Could you check a few things on this model? Use its own coordinates, in mm. A direction names the side the tool comes from. Give positions to 0.01 mm unless a question says otherwise; leave off trailing zeros. Order: outer loops, then holes, each group sorted by start corner. A loop starts at its lowest first (then second) coordinate and runs counter-clockwise, first axis right, second up. Notation, with made-up numbers: M 81.25,8 L 128.25,8 A32 ccw 128.25,37 Z; hole C 48,38 d6. An arc over 180 degrees is marked long. Use a Markdown table: item, result. Add a question column.
Item 1: I'm going to push flat-ended pins straight in: pin 1 Ø9 at (x, z) = (8, 5.5) entering from +Y; pin 2 Ø1 at (x, z) = (14, 11) entering from +Y; pin 3 Ø3.5 at (y, z) = (9.5, 13) entering from -X; pin 4 Ø8.5 at (x, z) = (8.5, 4) entering from -Y. Where does each tip first touch, or does it pass through?
Item 2: If I drill on L1, parallel to Y at x = 11, z = 3.25; L2, parallel to Z at x = 6, y = 9.75; L3, parallel to X at y = 2.75, z = 8.5, over which ranges is the centre line in solid material (lowest first)? Write a range as from..to.
Item 3: If we mould it in two halves opening along Y, with no side actions, what happens to faces 4 (the face through (6, 5, 27)), 5 (the face through (-0.25, 1, 13)), 6 (the face through (0, 6.65, 13))? For each: released by +Y, released by -Y, zero draft, split by the parting line, or undercut.
Item 4: For faces 1 (the face through (2.4, 7.22, 13.79)), 2 (the face through (6, 4.65, 13)), 3 (the face through (6, -2.15, 4)), which set-ups out of +Z, -Z, +X, -X, +Y, -Y let a thin tool reach every point of the face, with its end or its side?
Item 5: Suppose I cut it at D-D on z = 3.5. Write out the boundary of the cut face in (x, y).
Item 6: Suppose I cut it at A-A on x = 6. Write out the boundary of the cut face in (y, z), plus the area to 3 significant figures.
Item 7: Suppose I cut it at B-B on z = 23.5. Write out the boundary of the cut face in (x, y), plus the area to 3 significant figures.
Item 8: Suppose I cut it at C-C on y = 1.25. Write out the boundary of the cut face in (x, z).
from build123d import *

# Parameters (mm, degrees)
F0_W      = 12.5
F0_H      = 4.8
F1_DEPTH  = 27
F2_W      = 12.5
F2_H      = 6.8
F3_DEPTH  = 19
F4_W      = 1.5
F4_H      = 0.3
F5_DEPTH  = 3
F6_R      = 1.3
F7_DEPTH  = 13.801
F8_R      = 2
F10_DEPTH = 0.2


with BuildPart() as f1:
    # F0 (on Top) → F1 (new body)
    with BuildSketch(Plane.XY):
        Polygon((3, 6.65), (-2.25, 6.65), (-2.25, -2.15), (14.25, -2.15), (14.25, 6.65), (9, 6.65), (9, 11.65), (3, 11.65), align=None)
        with Locations((6, 2.25)):
            Rectangle(F0_W, F0_H, mode=Mode.SUBTRACT)
    extrude(amount=F1_DEPTH)

    # F2 (on face) → F3 (cut)
    with BuildSketch(Plane.XY.offset(27)):
        with Locations((6, 1.25)):
            Rectangle(F2_W, F2_H)
    extrude(amount=-F3_DEPTH, mode=Mode.SUBTRACT)

    # F4 (on face) → F5 (join)
    with BuildSketch(Plane.XY.offset(8)):
        with Locations((0.5, 0)):
            Rectangle(F4_W, F4_H)
        with Locations((11.5, 0)):
            Rectangle(F4_W, F4_H)
    extrude(amount=-F5_DEPTH)

    # F6 (on face) → F7 (cut, through all)
    with BuildSketch(Plane(origin=(0, 11.65, 0), x_dir=(-1, 0, 0), z_dir=(0, 1, 0))):
        with Locations((-6, 23.5)):
            Circle(F6_R)
    extrude(amount=-F7_DEPTH, mode=Mode.SUBTRACT)

    # F8
    f8_edges = [f1.edges().sort_by_distance(p)[0] for p in [
        (9, 6.65, 13.5),
        (3, 6.65, 13.5),
        (-2.25, 6.65, 13.5),
        (-2.25, -2.15, 13.5),
        (14.25, 6.65, 13.5),
        (14.25, -2.15, 13.5),
        (6, 11.65, 27),
    ]]
    fillet(f8_edges, radius=F8_R)

    # F9 (on face) → F10 (join)
    with BuildSketch(Plane(origin=(0, 0, 0), x_dir=(1, 0, 0), z_dir=(0, 0, -1))):
        with BuildLine():
            ThreePointArc((-0.25, 4.15), (-3.0784271247, 2.9784271247), (-4.25, 0.15))
            Line((-4.25, 0.15), (-4.25, -4.65))
            ThreePointArc((-4.25, -4.65), (-3.0784271247, -7.4784271247), (-0.25, -8.65))
            Line((-0.25, -8.65), (1, -8.65))
            Line((1, -8.65), (1, -11.65))
            ThreePointArc((1, -11.65), (1.5857864376, -13.0642135624), (3, -13.65))
            Line((3, -13.65), (9, -13.65))
            ThreePointArc((9, -13.65), (10.4142135624, -13.0642135624), (11, -11.65))
            Line((11, -11.65), (11, -8.65))
            Line((11, -8.65), (12.25, -8.65))
            ThreePointArc((12.25, -8.65), (15.0784271247, -7.4784271247), (16.25, -4.65))
            Line((16.25, -4.65), (16.25, 0.15))
            ThreePointArc((16.25, 0.15), (15.0784271247, 2.9784271247), (12.25, 4.15))
            Line((12.25, 4.15), (-0.25, 4.15))
        make_face()
        with BuildLine():
            ThreePointArc((-0.25, -6.65), (-1.6642135624, -6.0642135624), (-2.25, -4.65))
            Line((-2.25, -4.65), (-2.25, 0.15))
            ThreePointArc((-2.25, 0.15), (-1.6642135624, 1.5642135624), (-0.25, 2.15))
            Line((-0.25, 2.15), (12.25, 2.15))
            ThreePointArc((12.25, 2.15), (13.6642135624, 1.5642135624), (14.25, 0.15))
            Line((14.25, 0.15), (14.25, -4.65))
            ThreePointArc((14.25, -4.65), (13.6642135624, -6.0642135624), (12.25, -6.65))
            Line((12.25, -6.65), (11, -6.65))
            ThreePointArc((11, -6.65), (9.5857864376, -7.2357864376), (9, -8.65))
            Line((9, -8.65), (9, -11.65))
            Line((9, -11.65), (3, -11.65))
            Line((3, -11.65), (3, -8.65))
            ThreePointArc((3, -8.65), (2.4142135624, -7.2357864376), (1, -6.65))
            Line((1, -6.65), (-0.25, -6.65))
        make_face(mode=Mode.SUBTRACT)
    extrude(amount=-F10_DEPTH)


solid = f1.part
Findings below:
| question | item | result |
|---|---|---|
| 1 | pin 1 | stops at y = 11.65 |
| 1 | pin 2 | stops at y = 6.21 |
| 1 | pin 3 | stops at x = 2.79 |
| 1 | pin 4 | stops at y = -4.15 |
| 2 | L1 | y = -2.15..-0.15, 4.65..6.65 |
| 2 | L2 | z = 0..22.2, 24.8..27 |
| 2 | L3 | x = -2.25..-0.25, 12.25..14.25 |
| 3 | face 4 | zero draft |
| 3 | face 5 | undercut |
| 3 | face 6 | released by +Y |
| 4 | face 1 | +Z, -X, +Y |
| 4 | face 2 | +Z, -Z |
| 4 | face 3 | +Z, +X, -X, -Y |
| 5 | outline | M -2.25,-0.15 A2 ccw -0.25,-2.15 L 12.25,-2.15 A2 ccw 14.25,-0.15 L 14.25,4.65 A2 ccw 12.25,6.65 L 11,6.65 A2 cw 9,8.65 L 9,11.65 L 3,11.65 L 3,8.65 A2 cw 1,6.65 L -0.25,6.65 A2 ccw -2.25,4.65 Z; hole M -0.25,-0.15 L 12.25,-0.15 L 12.25,4.65 L -0.25,4.65 Z |
| 6 | outline | M -4.15,0 L -0.15,0 L -0.15,8 L -2.15,8 L -2.15,0.2 L -4.15,0.2 Z; M 4.65,0 L 13.65,0 L 13.65,0.2 L 11.65,0.2 L 11.65,22.2 L 4.65,22.2 Z; M 4.65,24.8 L 11.65,24.8 L 11.65,25 A2 ccw 9.65,27 L 4.65,27 Z |
| 6 | area | 187 mm^2 |
| 7 | outline | M -2.25,-0.15 A2 ccw -0.25,-2.15 L -0.25,4.65 L 4.7,4.65 L 4.7,11.65 L 3,11.65 L 3,8.65 A2 cw 1,6.65 L -0.25,6.65 A2 ccw -2.25,4.65 Z; M 7.3,4.65 L 12.25,4.65 L 12.25,-2.15 A2 ccw 14.25,-0.15 L 14.25,4.65 A2 ccw 12.25,6.65 L 11,6.65 A2 cw 9,8.65 L 9,11.65 L 7.3,11.65 Z |
| 7 | area | 70.3 mm^2 |
| 8 | outline | M -4.25,0 L -0.25,0 L -0.25,27 L -2.25,27 L -2.25,0.2 L -4.25,0.2 Z; M 12.25,0 L 16.25,0 L 16.25,0.2 L 14.25,0.2 L 14.25,27 L 12.25,27 Z |
